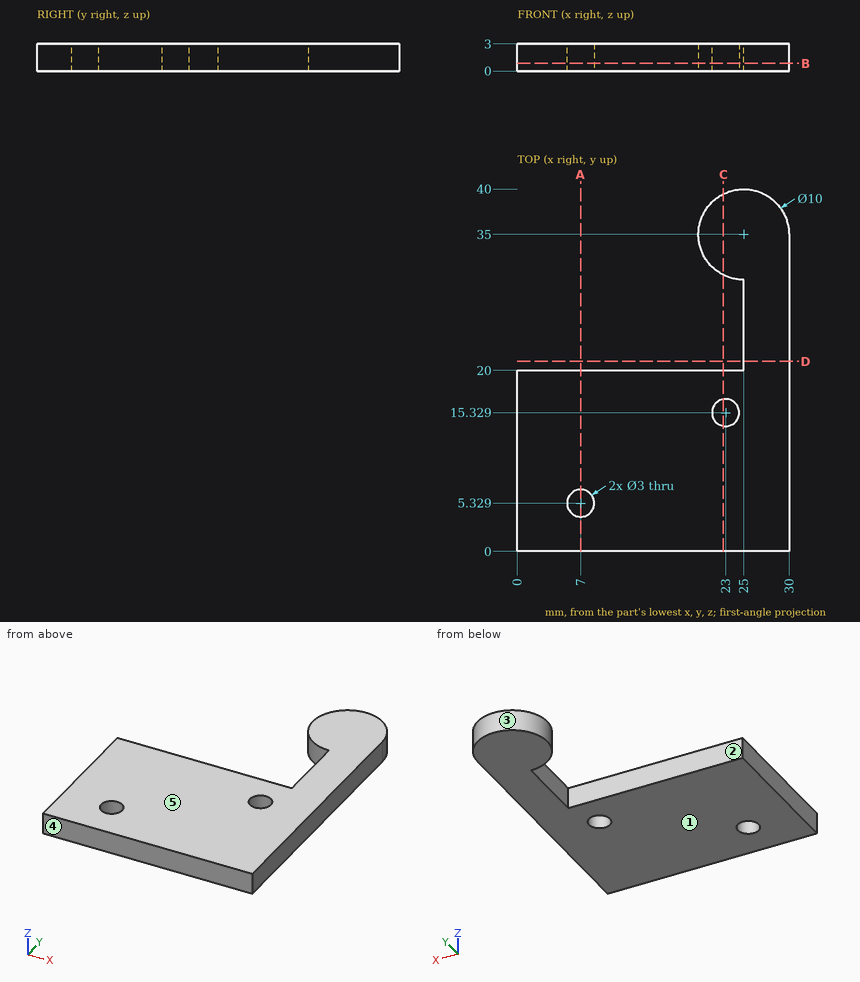
Answer from the drawing. Dimensions are ordinates in mm from the lowest x, y and z of the part. A direction names the side the tool comes from. Coordinates: 2 decimals unless noted, no trailing zeros. Order: outer loops, then holes, each group sorted by start corner. A loop starts at its lowest first (then second) coordinate and runs counter-clockwise, first axis right, second up. Notation, with made-up numbers: M 23.5,45 L 32.5,45 A12 ccw 32.5,55 Z; hole C -25,44 d6. An arc over 180 degrees is marked long. Put each result on its own line as item: value. Start each with the question number.
Item 1: Section D-D, the plane y = 21 is taken. Determine the outline of the cut face in (x, z), plus the area to 3 significant figures.
Item 2: The mould has two halves that part along Y. Classify the marked faces 3, 4 and 5: +Y half, -Y half, draft (parallel to the pull), parting line (faces both ways), or undercut.
Item 3: Section B-B, the plane z = 0.85 is taken. Determine the outline of the cut face in (x, y), plus the area to 3 significant figures.
Item 4: Given pin 1 Ø1 at (x, z) = (21, 1) entering from +Y; pin 2 Ø5 at (x, y) = (23, 15.33) entering from +Z; pin 3 Ø0.9 at (y, z) = (22.5, 1.5) entering from -X, each flat-ended and moving along its own axis, determine where each tip first touches the part or whether it passes through.
Item 5: Consider probe 1 along X at (y, z) = (24, 1.6); probe 2 along Y at (x, z) = (12.75, 2.65); probe 3 along Y at (x, z) = (7, 1.85). Determine where each line is inside the solid, lowest interval first. Write a range as [from, to].
Item 6: Section C-C, the plane x = 22.75 is taken. Count the separate pieces of the cut face and the enclosed holes in it.
Item 7: For the marked faces 1 and 2, determine the directions among +Z, -Z, +X, -X, +Y, -Y from which every point of the face is accessible in a straight line to the end or side of a thin tool.
Item 8: Section A-A, the plane x = 7 is taken. Determine the outline of the cut face in (y, z), plus the area to 3 significant figures.
Computed:
1. outline: M 25,0 L 30,0 L 30,3 L 25,3 Z
1. area: 15.0 mm2
2. face 3: undercut
2. face 4: -Y half
2. face 5: draft
3. outline: M 0,0 L 30,0 L 30,35 A5 ccw long 25,30 L 25,20 L 0,20 Z; hole C 7,5.33 d3; hole C 23,15.33 d3
3. area: 720 mm2
4. pin 1: stops at y = 38.57
4. pin 2: stops at z = 3
4. pin 3: stops at x = 25
5. probe 1: x = [25, 30]
5. probe 2: y = [0, 20]
5. probe 3: y = [0, 3.83], [6.83, 20]
6. separate pieces: 3
6. enclosed holes: 0
7. face 1: -Z, +X, -X, +Y, -Y
7. face 2: +Z, -Z, -X
8. outline: M 0,0 L 3.83,0 L 3.83,3 L 0,3 Z; M 6.83,0 L 20,0 L 20,3 L 6.83,3 Z
8. area: 51.0 mm2
